Autodesk Inventor part; units mm, degrees
ref_plane "YZ Plane" through (0, 0, 0) normal (1, 0, 0) x (0, 1, 0)
ref_plane "XZ Plane" through (0, 0, 0) normal (0, 1, 0) x (-1, 0, 0)
ref_plane "XY Plane" through (0, 0, 0) normal (0, 0, 1) x (1, 0, 0)
sketch "Sketch1" plane through (0, 0, 0) normal (0, 0, 1) x (1, 0, 0)
  line L0 (-34, 30) -> (-34, -100)
  line L1 (96, -68) -> (96, -24)
  line L2 (0, -10) -> (0, 30)
  line L3 (-10, 40) -> (-24, 40)
  circle A0 centre (78, -60) radius 1.3
  circle A1 centre (-7.65, 3.7) radius 1.3
  arc A2 (-24, 40) -> (-34, 30) centre (-24, 30) ccw
  arc A3 (0, 30) -> (-10, 40) centre (-10, 30) ccw
  arc A4 (86, -78) -> (96, -68) centre (86, -68) ccw
  line L4 (0, -82) -> (0, -100)
  line L5 (-10, -110) -> (-24, -110)
  arc A5 (-10, -110) -> (0, -100) centre (-10, -100) ccw
  arc A6 (-34, -100) -> (-24, -110) centre (-24, -100) ccw
  line L6 (59, -14) -> (86, -14)
  arc A7 (96, -24) -> (86, -14) centre (86, -24) ccw
  line L7 (54, -74) -> (54, -70)
  line L8 (50, -66) -> (13, -66)
  line L9 (9, -70) -> (9, -72)
  line L10 (5, -78) -> (4, -78)
  line L11 (58, -78) -> (86, -78)
  arc A8 (13, -66) -> (9, -70) centre (13, -70) ccw
  arc A9 (54, -74) -> (58, -78) centre (58, -74) ccw
  arc A10 (54, -70) -> (50, -66) centre (50, -70) ccw
  line L12 (-16.3182, -100.6212) -> (-22.7887, -76.473)
  line L13 (-22.7887, -76.473) -> (-20.4705, -75.8519)
  line L14 (-20.4705, -75.8519) -> (-14, -100)
  line L15 (-14, -100) -> (-16.3182, -100.6212)
  line L16 (-10, -100) -> (-24, -100) construction
  line L17 (-34, -35) -> (96, -35) construction
  line L18 (-15.5455, 32) -> (-23.8277, 1.0904)
  line L19 (-15.5455, 32) -> (-14, 31.5859)
  line L20 (-14, 31.5859) -> (-22.2822, 0.6763)
  line L21 (-22.2822, 0.6763) -> (-23.8277, 1.0904)
  line L22 (53, -20) -> (10, -20)
  line L23 (56, -17) -> (56, -17)
  arc A11 (53, -20) -> (56, -17) centre (53, -17) ccw
  arc A12 (59, -14) -> (56, -17) centre (59, -17) ccw
  arc A13 (0, -10) -> (10, -20) centre (10, -10) ccw
  line L24 (-10, 30) -> (-24, 30) construction
  circle A14 centre (60, -20) radius 1.3
  circle A15 centre (58, -72) radius 1.3
  line L25 (9, -72) -> (9, -74)
  arc A16 (5, -78) -> (9, -74) centre (5, -74) ccw
  arc A17 (4, -78) -> (0, -82) centre (4, -82) ccw
  circle A18 centre (-8, -72) radius 1.3
  line L26 (58, -72) -> (-8, -72) construction
  point P0 (0, 0)
  point P1 (-34, 40)
  point P2 (0, 40)
  point P3 (-34, -110)
  point P4 (96, -14)
  point P5 (9, -78)
  point P6 (0, -20)
  point P7 (54, -66)
  point P8 (9, -66)
  dimension "d2" = 2.6
  dimension "d4" = 18
  dimension "d5" = 40
  dimension "d7" = 34
  dimension "d10" = 26.35
  dimension "d14" = 10
  dimension "d23" = 10
  dimension "d25" = 17.7
  dimension "d27" = 45
  dimension "d29" = 64
  dimension "d31" = 32
  dimension "d32" = 12
  dimension "d33" = 130
  dimension "d36" = 4
  dimension "d38" = 2.4
  dimension "d39" = 75
  dimension "d42" = 42
  dimension "d46" = 1.6
  dimension "d48" = 6
  dimension "d49" = 3
  dimension "d50" = 10
  dimension "d51" = 75
  dimension "d52" = 32
  dimension "d55" = 8
  dimension "d56" = 14
  dimension "d57" = 25
  dimension "d58" = 14
  dimension "d59" = 40
  dimension "d60" = 18
  dimension "d61" = 20
  dimension "d62" = 12
  dimension "d63" = 20
  dimension "d64" = 100
  dimension "d65" = 4
  dimension "d66" = 60
  dimension "d67" = 4
  dimension "d68" = 66
extrude "Extrusion1" add sketch "Sketch1" along normal blind 3.175
properties part number "battery_mount"
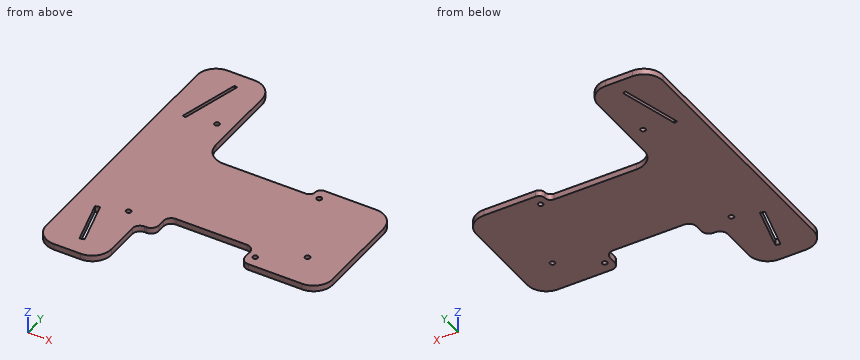
Geometry check sheet. Reference: the model listing, model coordinates, mm. Give positions to 0.01 mm unless a question says otherwise; leave off trailing zeros. Loops run counter-clockwise (first coordinate to the right, second up) from the corner with the lowest first, then second, coordinate; pieces in that order, holes last. Notation, with made-up numbers: M -38,-37 L -7,-37 A17 ccw -7,-12 Z; hole C -27.5,-31.75 d5. An arc over 180 degrees is marked long. Answer as CSV lines item,"result".
Item 1: Cross-section at D-D on x = 63.5. Record the cut outline in (y, z) (3 decimals).
Values:
outline,"M -78,0 L -14,0 L -14,3.175 L -78,3.175 Z"
Item 2: Material ranges on line 1 (Y direction, x = -8, z = 1.1); line 2 (X direction, y = -72, z = 0.9); line 3 (Y direction, x = 60, z = 1.9), recorded low to high.
Values:
line 1,"y = -109.8 to -73.3, -70.7 to 2.45, 4.95 to 39.8"
line 2,"x = -34 to -9.3, -6.7 to 9, 54 to 56.7, 59.3 to 95.17"
line 3,"y = -78 to -21.3, -18.7 to -14"
Item 3: Cross-section at B-B on z = 1.05. Count the separate pieces of the cut face and the enclosed holes in it, and give its area (3 significant figures).
Values:
separate pieces,"1"
enclosed holes,"7"
area,"10,100 mm²"
Item 4: Cross-section at A-A on y = 22. Record the cut outline in (x, z) (3 decimals), and give its area (3 significant figures).
Values:
outline,"M -34,0 L -18.225,0 L -18.225,3.175 L -34,3.175 Z; M -16.569,0 L 0,0 L 0,3.175 L -16.569,3.175 Z"
area,"103 mm²"
Item 5: Depth check by flat-ended pin: P1, Ø1, axis at y = -11, z = 1, coming from the +X side; P2, Ø1.6, axis at x = 58, y = -72, coming from the -Z side; P3, Ø1, axis at y = -72, z = 1, coming from the +X side; P4, Ø0.5, axis at x = 4.5, z = 1, coming from the -Y side. Enter the tip coordinate at first touch or a pass-through.
Values:
P1,"stops at x = 0.11"
P2,"passes through"
P3,"stops at x = 95.37"
P4,"stops at y = -78"
Item 6: Cross-section at C-C on x = 28. Record the cut outline in (y, z) (3 decimals).
Values:
outline,"M -66,0 L -20,0 L -20,3.175 L -66,3.175 Z"
